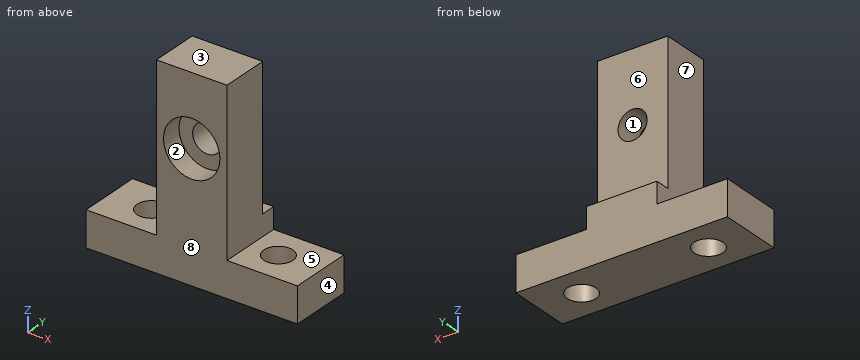
Autodesk Inventor part; units mm, degrees
ref_plane "YZ Plane" through (0, 0, 0) normal (1, 0, 0) x (0, 1, 0)
ref_plane "XZ Plane" through (0, 0, 0) normal (0, 1, 0) x (-1, 0, 0)
ref_plane "XY Plane" through (0, 0, 0) normal (0, 0, 1) x (1, 0, 0)
sketch "Sketch1" plane through (0, 0, 0) normal (0, 0, 1) x (1, 0, 0)
  line L0 (15, 0) -> (-15, 0)
  line L1 (-15, 0) -> (-15, 9)
  line L2 (-15, 9) -> (15, 9)
  line L3 (15, 9) -> (15, 0)
  line L4 (0, 10.8) -> (0, -1.8)
  circle A0 centre (9, 4.5) radius 2.0625
  circle A1 centre (-9, 4.5) radius 2.0625
  point P0 (0, 0)
  dimension "d0" = 9
  dimension "d1" = 30
  dimension "d4" = 4.125
  dimension "d5" = 6
  dimension "d6" = 4.5
extrude "Extrusion1" add sketch "Sketch1" along normal blind 5
sketch "Sketch2" plane through (0, 0, 5) normal (0, 0, 1) x (1, 0, 0)
  line L0 (-15, 0) -> (15, 0)
  line L1 (15, 9) -> (-15, 9)
  line L2 (5, 0) -> (-5, 0)
  line L3 (-5, 0) -> (-5, 9)
  line L4 (-5, 9) -> (5, 9)
  line L5 (5, 9) -> (5, 0)
  line L6 (0, 10.8) -> (0, -1.8)
  point P0 (0, 0)
  dimension "d7" = 10
extrude "Extrusion2" add sketch "Sketch2" along normal blind 3
sketch "Sketch3" plane through (0, 0, 8) normal (0, 0, 1) x (1, 0, 0)
  line L0 (-5, 9) -> (-5, 0)
  line L1 (5, 0) -> (-5, 0)
  line L2 (-5, 0) -> (-5, 6.9)
  line L3 (-5, 6.9) -> (5, 6.9)
  line L4 (5, 6.9) -> (5, 0)
  point P0 (0, 0)
  dimension "d10" = 6.9
extrude "Extrusion3" add sketch "Sketch3" along normal blind 20
sketch "Sketch4" plane through (-15, 0, 0) normal (0, -1, 0) x (1, 0, 0)
  circle A0 centre (15, 18) radius 4
  circle A1 centre (15, 18) radius 2.0625
  line L0 (10, 28) -> (20, 28)
  point P0 (15, 0)
  dimension "d13" = 8
  dimension "d14" = 4.125
  dimension "d19" = 10
extrude "Extrusion4" cut sketch "Sketch4" against normal blind 3 contours A0 | A1
extrude "Extrusion5" cut sketch "Sketch4" against normal up to next contours A1
properties part number "Linear Bearing Adapter Arm"
Geometry: final body of the model. Coordinates: model frame, mm. Face numbers are marked on the shaded views. A direction names the side the tool comes from. Round coordinates to 2 decimals unless told otherwise and drop trailing zeros. Order: outer loops, then holes, each group sorted by start corner. A loop starts at its lowest first (then second) coordinate and runs counter-clockwise, first axis right, second up. Notation, with made-up numbers: M -4.75,-29.5 L 18.25,-29.5 A31 cw 18.25,1.5 Z; hole C 55.25,51.25 d5. An arc over 180 degrees is marked long. One line per item, written item: value.
(1) Cut plane D-D (z = 3.5). Return the cut outline in (x, y) (1 decimal).
Result sheet:
outline: M -15,0 L 15,0 L 15,9 L -15,9 Z; hole C -9,4.5 d4.1; hole C 9,4.5 d4.1
(2) Cut plane B-B (y = 5.5). Return the cut outline in (x, z) (1 decimal).
Result sheet:
outline: M -15,0 L -10.8,0 L -10.8,5 L -15,5 Z; M -7.2,0 L 7.2,0 L 7.2,5 L 5,5 L 5,28 L -5,28 L -5,5 L -7.2,5 Z; M 10.8,0 L 15,0 L 15,5 L 10.8,5 Z; hole C 0,18 d4.1
(3) Reachability of the marked faces 5, 6, 7 and 8 from +Z, -Z, +X, -X, +Y, -Y: full face, straight path, thin tool, end or side. Return the list, or none.
Result sheet:
face 5: +Z, +X, +Y, -Y
face 6: +Z, +X, -X, +Y
face 7: +Z, -X, +Y, -Y
face 8: +Z, -Z, +X, -X, -Y
(4) Pin query (flat end, axial travel): P1, Ø2, axis at x = 7, y = 7.5, coming from the +Z side; P2, Ø4.5, axis at x = -9, y = 4.5, coming from the -Z side; P3, Ø5.5, axis at x = 0, z = 18, coming from the -Y side; P4, Ø5, axis at x = -1, z = 20.5, coming from the +Y side. Return the tip coordinate at first contact, or that it passes through.
Result sheet:
P1: z = 5
P2: z = 0
P3: y = 3
P4: y = 6.9
(5) Pull-direction query (Z, two-part tool) for the marked faces 1, 2, 3 and 4; classes: pulls with the +Z half, pulls with the -Z half, needs draft (parallel to the pull), parting line crosses it, or undercut.
Result sheet:
face 1: undercut
face 2: undercut
face 3: pulls with the +Z half
face 4: needs draft
(6) Line query: probe 1 along Y at (x, z) = (-9, 2); probe 2 along Z at (x, y) = (10, 1.5); probe 3 along Z at (x, y) = (0, 2.1). Output: solid intervals per line, ascending. Write a range as [from, to].
Result sheet:
probe 1: [0, 2.44], [6.56, 9]
probe 2: [0, 5]
probe 3: [0, 14], [22, 28]
(7) Cut plane C-C (z = 18). Return the cut outline in (x, y).
Result sheet:
outline: M -5,0 L -4,0 L -4,3 L -2.06,3 L -2.06,6.9 L -5,6.9 Z; M 2.06,3 L 4,3 L 4,0 L 5,0 L 5,6.9 L 2.06,6.9 Z
(8) Cut plane A-A (x = 0). Return the cut outline in (y, z), and give its area (3 significant figures).
Result sheet:
outline: M 0,0 L 9,0 L 9,8 L 6.9,8 L 6.9,15.94 L 3,15.94 L 3,14 L 0,14 Z; M 0,22 L 3,22 L 3,20.06 L 6.9,20.06 L 6.9,28 L 0,28 Z
area: 170 mm2
